Read the model definition and answer for the solid it produces. Units are mm, in the model's axes. A direction names the side the tool comes from. Round coordinates to 2 decimals unless told otherwise and drop trailing zeros. Order: outer loops, then holes, each group sorted by start corner. A loop starts at its lowest first (then second) coordinate and runs counter-clockwise, first axis right, second up. Notation, with made-up numbers: (88, -19) - (109, -19) arc R8 ccw to (109, -6) - close; hole circle Ø2 at (60.25, 70.5). An arc over 180 degrees is marked (long way). Put each result on its own line as item: value. Start each with the question number.
Q1. Section C-C on x = -5.5 is taken. Give the vertices of the cut face in (y, z) (1 decimal).
Q2. Each of these flat-tipped pins is pushed along its axis until it touches: pin 1 Ø4 at (x, y) = (-4.5, 1) entering from -Z; pin 2 Ø5 at (y, z) = (8.5, 2.5) entering from +X; pin 3 Ø2 at (x, z) = (5, 2) entering from -Y. Where does it stop, or does it pass through?
Q3. Find the intervals of material crossed by line 1 along Y through (x, z) = (0, 12); line 2 along Z through (x, y) = (7, 20); line 3 along X through (y, z) = (0, 12.2), in increasing order. Write a range as from..to.
Q4. Which of the six approach directions +Z, -Z, +X, -X, +Y, -Y give full straight-line access (tool end or side, diameter ignored) to faces 1 (the face through (0, 12, 4)), 2 (the face through (-8, 19, 9))?
Q5. Section D-D on z = 9.5 is taken. Give the vertices of the cut face in (x, y) (1 decimal).
Q6. For a pull along X with two mould halves and no side action, classify faces 3 (the face through (8, 18, 9)), 4 (the face through (-0.54, -2.44, 11.99)), 5 (the face through (-6.22, 21.574, 7.707)), 6 (the face through (-4.4, 18.18, 7.4)) as pulls with the +X half, pulls with the -X half, needs draft (parallel to the pull), parting line crosses it, or undercut.
Q7. Section B-B on y = 20 is taken. Give the vertices of the cut face in (x, z).
Q8. Section A-A on z = 7.5 is taken. Give the vertices of the cut face in (x, y) (1 decimal).
from build123d import *

# Parameters (mm, degrees)
SKETCH1_R                  = 2.5
BOSS_EXTRUDE1_DEPTH        = 15
SKETCH6_W                  = 16
SKETCH6_H                  = 20
CUT_EXTRUDE1_DEPTH         = 9
FILLET1_R                  = 2.5
F_3_8_0_3750_DOWEL_HOLE1_D = 9.525
F_1_8_0_1250_DOWEL_HOLE1_D = 3.175


with BuildPart() as part:
    # Sketch1 → Boss-Extrude1 (new body)
    with BuildSketch(Plane.XY):
        with BuildLine():
            Line((-8, 12), (-8, 0))
            ThreePointArc((-8, 0), (0, -8), (8, 0))
            Line((8, 0), (8, 12))
            Line((8, 12), (8, 30))
            Line((8, 30), (-8, 30))
            Line((-8, 30), (-8, 12))
        make_face()
        Circle(SKETCH1_R, mode=Mode.SUBTRACT)
    extrude(amount=BOSS_EXTRUDE1_DEPTH)

    # Sketch6 → Cut-Extrude1 (cut)
    with BuildSketch(Plane.XY):
        with Locations((0, 2)):
            Rectangle(SKETCH6_W, SKETCH6_H)
    extrude(amount=CUT_EXTRUDE1_DEPTH, mode=Mode.SUBTRACT)

    # Fillet1
    fillet1_edges = [part.edges().sort_by_distance(p)[0] for p in [
        (-2.5, 0, 15),
        (-2.5, 0, 9),
    ]]
    fillet(fillet1_edges, radius=FILLET1_R)

    # 3/8 (0.3750) Dowel Hole1 (through all)
    with Locations(Plane.XY.offset(15)):
        with Locations((0, 20)):
            Hole(F_3_8_0_3750_DOWEL_HOLE1_D / 2)

    # 1/8 (0.1250) Dowel Hole1 (through all)
    with Locations(Plane.ZY.offset(8)):
        with Locations((7.5, 20)):
            Hole(F_1_8_0_1250_DOWEL_HOLE1_D / 2)


solid = part.part
Findings:
1. outline: (-5.8, 9) - (12, 9) - (12, 0) - (30, 0) - (30, 15) - (-5.8, 15) - close; hole circle Ø3.2 at (20, 7.5)
2. pin 1: z = 9
2. pin 2: through
2. pin 3: y = 12
3. line 1: -8..-2.5, 2.5..15.24, 24.76..30
3. line 2: 0..5.91, 9.09..15
3. line 3: -8..-2.5, 2.5..8
4. face 1: -Z, +X, -X, -Y
4. face 2: +Z, -Z, -X, +Y, -Y
5. outline: (-8, 0) arc R8 ccw to (8, 0) - (8, 30) - (-8, 30) - close; hole circle Ø9.5 at (0, 20); hole circle Ø7 at (0, 0)
6. face 3: pulls with the +X half
6. face 4: undercut
6. face 5: needs draft
6. face 6: undercut
7. outline: (-8, 0) - (-4.76, 0) - (-4.76, 5.91) - (-8, 5.91) - close; (-8, 9.09) - (-4.76, 9.09) - (-4.76, 15) - (-8, 15) - close; (4.76, 0) - (8, 0) - (8, 5.91) - (4.76, 5.91) - close; (4.76, 9.09) - (8, 9.09) - (8, 15) - (4.76, 15) - close
8. outline: (-8, 12) - (8, 12) - (8, 18.4) - (4.5, 18.4) arc R4.8 cw to (-4.5, 18.4) - (-8, 18.4) - close; (-8, 21.6) - (-4.5, 21.6) arc R4.8 cw to (4.5, 21.6) - (8, 21.6) - (8, 30) - (-8, 30) - close
